For this review, use the dimensioned drawing (mm, ordinates from the lowest corner) and the shaded views. A direction names the side the tool comes from. Coordinates: 2 decimals unless noted, no trailing zeros. Write each loop counter-clockwise with the first axis right and the second up, starting at its lowest first coordinate (ties: lowest second). Pieces come first, ordered by that corner, then holes. Notation, with made-up numbers: (-14, 42) - (17, 42) arc R19 cw to (17, 51) - close; hole circle Ø8 at (-2.75, 64). An arc over 180 degrees is marked (long way). Answer as a JSON object with one key per item and string values.
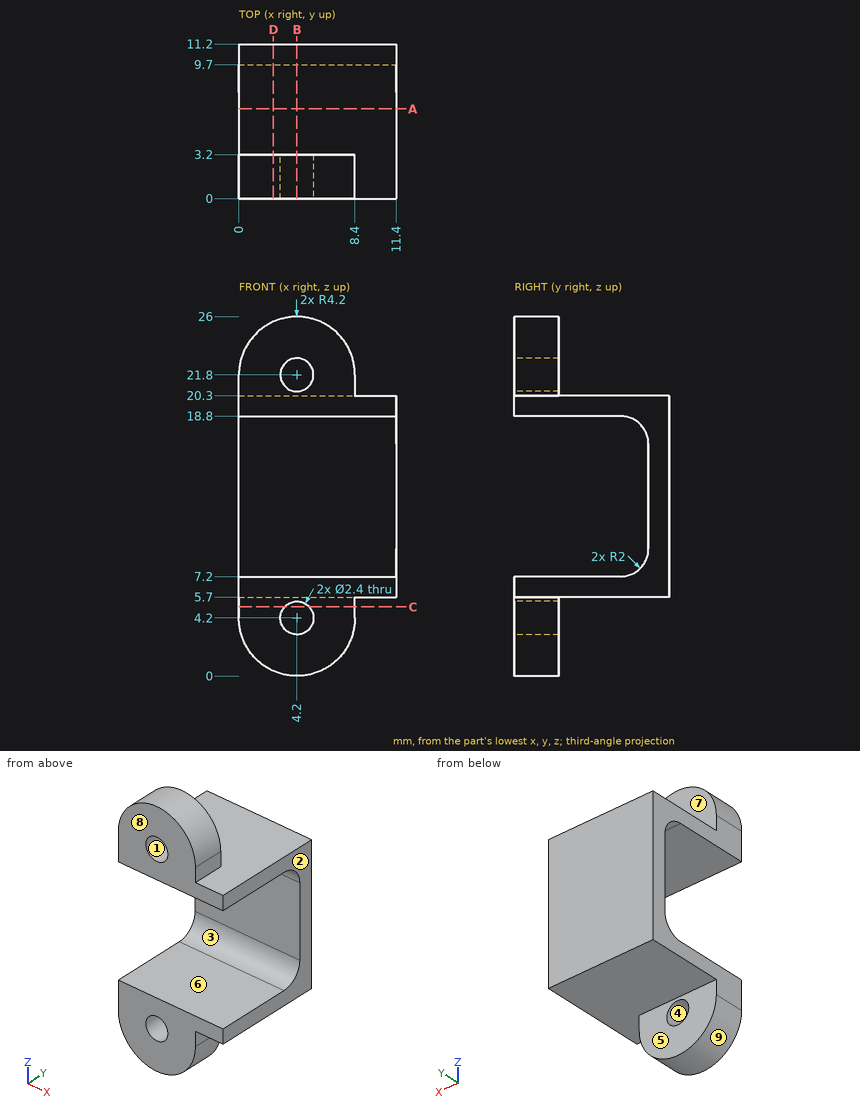
(1) To check wall thickness, follow line 1 (Z direction, x = 4.2, y = 0.85); line 2 (Z direction, x = 10.5, y = 2); line 3 (X direction, y = 0.7, z = 21.8). State the ranges of each line that lie inside material, in increasing order. Write a range as from..to.
Solved:
{"line 1": "z = 0..3, 5.4..7.2, 18.8..20.6, 23..26", "line 2": "z = 5.7..7.2, 18.8..20.3", "line 3": "x = 0..3, 5.4..8.4"}
(2) Take a section at A-A, the plane y = 6.5. Write out the cut boundary in (x, z).
Solved:
{"outline": "(0, 5.7) - (11.4, 5.7) - (11.4, 7.2) - (0, 7.2) - close; (0, 18.8) - (11.4, 18.8) - (11.4, 20.3) - (0, 20.3) - close"}
(3) Take a section at B-B, the plane x = 4.2. Write out the cut boundary in (y, z).
Solved:
{"outline": "(0, 0) - (3.2, 0) - (3.2, 3) - (0, 3) - close; (0, 5.4) - (3.2, 5.4) - (3.2, 5.7) - (11.2, 5.7) - (11.2, 20.3) - (3.2, 20.3) - (3.2, 20.6) - (0, 20.6) - (0, 18.8) - (7.7, 18.8) arc R2 cw to (9.7, 16.8) - (9.7, 9.2) arc R2 cw to (7.7, 7.2) - (0, 7.2) - close; (0, 23) - (3.2, 23) - (3.2, 26) - (0, 26) - close"}
(4) Take a section at D-D, the plane x = 2.5. Write out the cut boundary in (y, z), and give its area (3 significant figures).
Solved:
{"outline": "(0, 0.36) - (3.2, 0.36) - (3.2, 5.7) - (11.2, 5.7) - (11.2, 20.3) - (3.2, 20.3) - (3.2, 25.64) - (0, 25.64) - (0, 18.8) - (7.7, 18.8) arc R2 cw to (9.7, 16.8) - (9.7, 9.2) arc R2 cw to (7.7, 7.2) - (0, 7.2) - close", "area": "86.9 mm^2"}
(5) Take a section at C-C, the plane z = 5. Write out the cut boundary in (x, y), and give its area (3 significant figures).
Solved:
{"outline": "(0, 0) - (3.31, 0) - (3.31, 3.2) - (0, 3.2) - close; (5.09, 0) - (8.4, 0) - (8.4, 3.2) - (5.09, 3.2) - close", "area": "21.2 mm^2"}
(6) Tool access review of the marked faces 5, 6, 7, 8 and 9: name each direction out of +Z, -Z, +X, -X, +Y, -Y from which nothing blocks a thin tool from reaching the whole face with its end or side.
Solved:
{"face 5": "-Z, +X, -X, +Y", "face 6": "+X, -X, -Y", "face 7": "+Z, +X, -X, +Y", "face 8": "+Z, -Z, +X, -X, -Y", "face 9": "-Z, +Y, -Y"}
(7) The part is to be moulded in two halves that separate along X. For the marked faces 1, 2, 3 and 4, say which applies: pulls with the +X half, pulls with the -X half, needs draft (parallel to the pull), parting line crosses it, or undercut.
Solved:
{"face 1": "undercut", "face 2": "pulls with the +X half", "face 3": "needs draft", "face 4": "undercut"}
(8) For pin 1 (2 mm diameter, centred on x = 9, y = 10, fed in from +Z); pin 2 (1.7 mm diameter, centred on x = 5, z = 3.5, fed in from +Y); pin 3 (3 mm diameter, centred on x = 1.5, y = 8.5, fed in from -Z), all flat-tipped, find the tip position at first contact; note any pin that passes through.
Solved:
{"pin 1": "stops at z = 20.3", "pin 2": "stops at y = 3.2", "pin 3": "stops at z = 5.7"}
